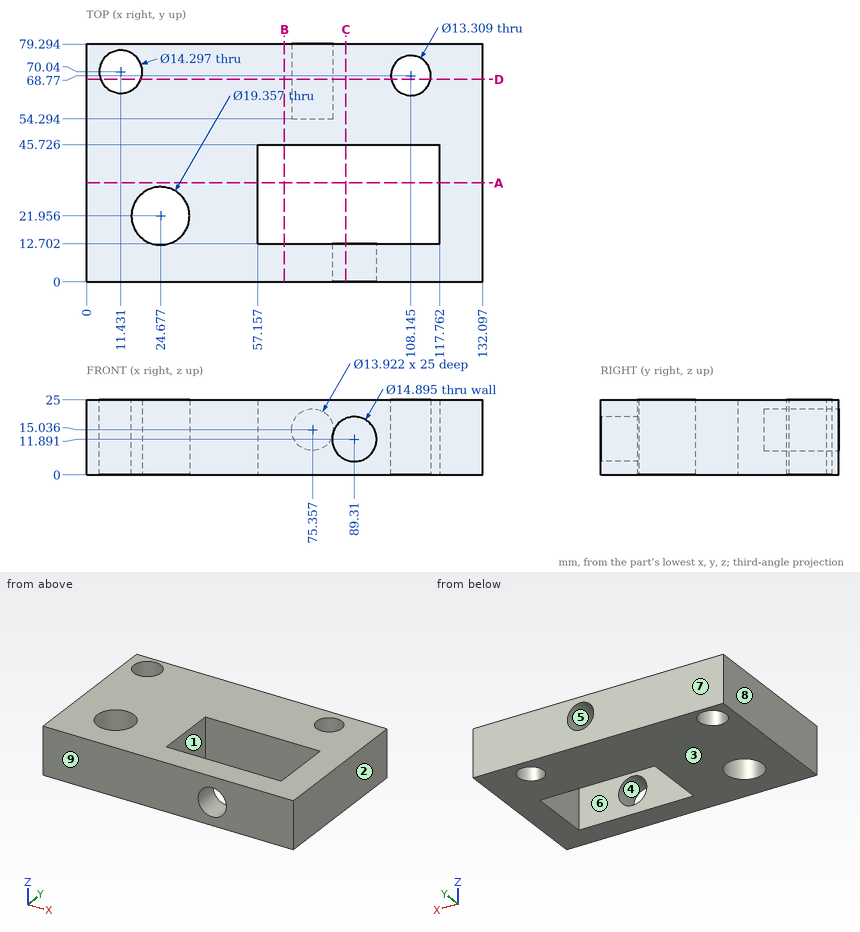
For this review, use the dimensioned drawing (mm, ordinates from the lowest corner) and the shaded views. A direction names the side the tool comes from. Give positions to 0.01 mm unless a question says otherwise; leave off trailing zeros. Order: outer loops, then holes, each group sorted by start corner. A loop starts at its lowest first (then second) coordinate and runs counter-clockwise, first axis right, second up.
1. Add section C-C, the plane x = 86.5. State the section outline as (y, z) points (1 decimal).
Solution:
outline: (0, 0) - (12.7, 0) - (12.7, 5) - (0, 5) - close; (0, 18.8) - (12.7, 18.8) - (12.7, 25) - (0, 25) - close; (45.7, 0) - (79.3, 0) - (79.3, 25) - (45.7, 25) - close
2. Tool access review of the marked faces 1, 2, 3, 4 and 5: name each direction out of +Z, -Z, +X, -X, +Y, -Y from which nothing blocks a thin tool from reaching the whole face with its end or side.
Solution:
face 1: +Z, -Z
face 2: +Z, -Z, +X, +Y, -Y
face 3: -Z, +X, -X, +Y, -Y
face 4: -Y
face 5: +Y
3. Add section D-D, the plane y = 67.5. State how many separate pieces and enclosed holes the cut face has, then the cut area to 3 significant figures.
Solution:
separate pieces: 3
enclosed holes: 1
area: 2,490 mm2
4. Add section A-A, the plane y = 33. State the section outline as (x, z) points, then the cut area to 3 significant figures.
Solution:
outline: (0, 0) - (57.16, 0) - (57.16, 25) - (0, 25) - close; (117.76, 0) - (132.1, 0) - (132.1, 25) - (117.76, 25) - close
area: 1,790 mm2
5. To check wall thickness, follow L1, parallel to X at y = 32, z = 14.5; L2, parallel to Y at x = 74.5, z = 2 (1 decimal); L3, parallel to X at y = 30, z = 18.5 (1 decimal). State the ranges of each line that lie inside material, in increasing order.
Solution:
L1: x = 0 to 57.16, 117.76 to 132.1
L2: y = 0 to 12.7, 45.7 to 79.3
L3: x = 0 to 19.3, 30.1 to 57.2, 117.8 to 132.1
6. For pin 1 Ø4 at (x, z) = (72, 14.5) entering from +Y; pin 2 Ø12 at (x, z) = (89.31, 11.89) entering from -Y, all flat-tipped, find the tip position at first contact; note any pin that passes through.
Solution:
pin 1: stops at y = 54.29
pin 2: stops at y = 45.73
7. Mouldability with a two-part tool opening along Y and no side actions: class the marked faces 6, 7, 8 and 9 as +Y half, -Y half, draft (parallel to the pull), parting line (faces both ways), or undercut.
Solution:
face 6: undercut
face 7: +Y half
face 8: draft
face 9: -Y half
8. Add section B-B, the plane x = 66. State the section outline as (y, z) points (1 decimal).
Solution:
outline: (0, 0) - (12.7, 0) - (12.7, 25) - (0, 25) - close; (45.7, 0) - (79.3, 0) - (79.3, 25) - (45.7, 25) - close
